Geometry: final body of the model. Coordinates: model frame, mm. Coordinates: 2 decimals unless noted, no trailing zeros. Order: outer loops, then holes, each group sorted by start corner. A loop starts at its lowest first (then second) coordinate and runs counter-clockwise, first axis right, second up. Notation, with made-up numbers: (-24, 12.5) -> (-12, 12.5) arc R26 ccw to (-12, 39.5) -> close; hole circle Ø11 at (-26, 26.25). An arc over 180 degrees is marked (long way). Use one line per item in the form item = value.
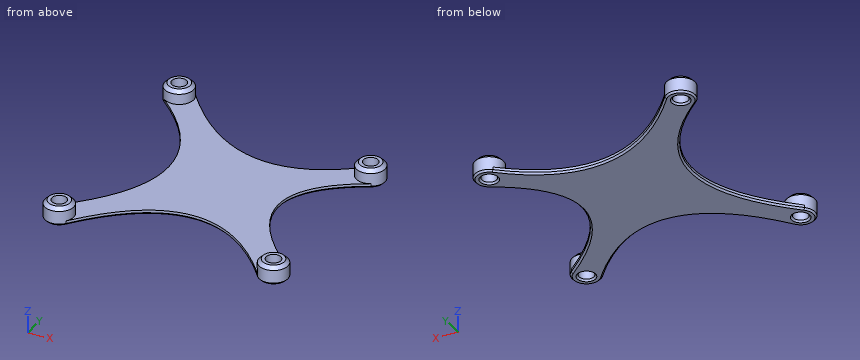
Autodesk Inventor part; units mm, degrees
ref_plane "YZ Plane" through (0, 0, 0) normal (1, 0, 0) x (0, 1, 0)
ref_plane "XZ Plane" through (0, 0, 0) normal (0, 1, 0) x (-1, 0, 0)
ref_plane "XY Plane" through (0, 0, 0) normal (0, 0, 1) x (1, 0, 0)
sketch "Skizze1" plane through (0, 0, 0) normal (0, 0, 1) x (1, 0, 0)
  circle A0 centre (-25.837, 27.4295) radius 1.65
  line L0 (-38.2086, 5.3216) -> (-37.4869, 5.3204)
  line L1 (-37.4869, 5.3204) -> (-37.4918, 2.4829)
  line L2 (-37.4918, 2.4829) -> (-35.7716, 2.4799)
  line L3 (-35.7716, 2.4799) -> (-35.7668, 5.1987)
  line L4 (-35.7668, 5.1987) -> (-35.0451, 5.1975)
  line L5 (-35.0451, 5.1975) -> (-35.0499, 2.4787)
  line L6 (-35.0499, 2.4787) -> (-32.1136, 2.4735)
  line L7 (-32.1136, 2.4735) -> (-32.115, 1.6628)
  line L8 (-32.115, 1.6628) -> (-38.215, 1.6735)
  line L9 (-38.215, 1.6735) -> (-38.2086, 5.3216)
  line L10 (-35.0952, -3.6509) -> (-32.1243, -3.6561)
  line L11 (-32.1243, -3.6561) -> (-32.1256, -4.4273)
  line L12 (-32.1256, -4.4273) -> (-34.7356, -4.4227)
  spline S0 degree 2 poles (-34.7356, -4.4227) (-35.052, -4.4222) (-35.5959, -4.4805) (-35.7592, -4.5692) knots 0 0 0 1 2 2 2
  spline S1 degree 2 poles (-35.7592, -4.5692) (-35.9323, -4.6628) (-36.101, -4.9987) (-36.1015, -5.2854) knots 0 0 0 1 2 2 2
  spline S2 degree 2 poles (-36.1015, -5.2854) (-36.102, -5.5721) (-35.7966, -6.1807) (-35.5499, -6.4728) knots 0 0 0 1 2 2 2
  line L13 (-35.5499, -6.4728) -> (-32.1292, -6.4787)
  line L14 (-32.1292, -6.4787) -> (-32.1305, -7.2499)
  line L15 (-32.1305, -7.2499) -> (-36.708, -7.2419)
  line L16 (-36.708, -7.2419) -> (-36.7066, -6.4707)
  line L17 (-36.7066, -6.4707) -> (-36.1975, -6.4716)
  spline S3 degree 2 poles (-36.1975, -6.4716) (-36.5083, -6.125) (-36.8334, -5.4571) (-36.8327, -5.0815) knots 0 0 0 1 2 2 2
  spline S4 degree 2 poles (-36.8327, -5.0815) (-36.8316, -4.4092) (-35.9405, -3.6495) (-35.0952, -3.6509) knots 0 0 0 1 2 2 2
  line L18 (-36.71, -8.3739) -> (-32.1325, -8.3819)
  line L19 (-32.1325, -8.3819) -> (-32.1338, -9.153)
  line L20 (-32.1338, -9.153) -> (-36.7113, -9.145)
  line L21 (-36.7113, -9.145) -> (-36.71, -8.3739)
  line L22 (-32.1384, -11.773) -> (-32.1398, -12.5837)
  line L23 (-32.1398, -12.5837) -> (-37.5181, -12.5743)
  line L24 (-37.5181, -12.5743) -> (-37.5217, -14.6208)
  line L25 (-37.5217, -14.6208) -> (-38.2434, -14.6195)
  line L26 (-38.2434, -14.6195) -> (-38.2348, -9.7158)
  line L27 (-38.2348, -9.7158) -> (-37.5131, -9.7171)
  line L28 (-37.5131, -9.7171) -> (-37.5167, -11.7636)
  line L29 (-37.5167, -11.7636) -> (-32.1384, -11.773)
  line L30 (-38.2719, -8.3168) -> (-37.4711, -8.3182)
  line L31 (-37.4711, -8.3182) -> (-37.4727, -9.1931)
  line L32 (-37.4727, -9.1931) -> (-38.2735, -9.1917)
  line L33 (-38.2735, -9.1917) -> (-38.2719, -8.3168)
  line L34 (-36.695, 0.2274) -> (-36.6936, 1.0282)
  line L35 (-36.6936, 1.0282) -> (-30.4347, -1.4445)
  line L36 (-30.4347, -1.4445) -> (-30.4362, -2.27)
  line L37 (-30.4362, -2.27) -> (-32.3428, -1.4461)
  line L38 (-32.3428, -1.4461) -> (-36.7008, -3.0994)
  line L39 (-36.7008, -3.0994) -> (-36.6993, -2.269)
  line L40 (-36.6993, -2.269) -> (-33.306, -1.0242)
  line L41 (-33.306, -1.0242) -> (-36.695, 0.2274)
  line L42 (-32.103, 8.529) -> (-32.5874, 8.5299)
  spline S5 degree 2 poles (-32.5874, 8.5299) (-32.5184, 8.4358) (-32.2718, 8.119) (-32.1979, 7.9706) knots 0 0 0 1 2 2 2
  spline S6 degree 2 poles (-32.1979, 7.9706) (-32.0895, 7.7677) (-31.9765, 7.3869) (-31.9771, 7.0409) knots 0 0 0 1 2 2 2
  spline S7 degree 2 poles (-31.9771, 7.0409) (-31.9775, 6.7591) (-32.191, 6.2503) (-32.3841, 6.0579) knots 0 0 0 1 2 2 2
  spline S8 degree 2 poles (-32.3841, 6.0579) (-32.5723, 5.8753) (-33.1263, 5.6538) (-33.4328, 5.6544) knots 0 0 0 1 2 2 2
  spline S9 degree 2 poles (-33.4328, 5.6544) (-33.9074, 5.6552) (-34.5789, 6.0568) (-34.771, 6.4921) knots 0 0 0 1 2 2 2
  spline S10 degree 2 poles (-34.771, 6.4921) (-34.9483, 6.878) (-35.0799, 7.9262) (-35.1134, 8.5343) knots 0 0 0 1 2 2 2
  line L43 (-35.1134, 8.5343) -> (-35.2617, 8.5345)
  spline S11 degree 2 poles (-35.2617, 8.5345) (-35.5287, 8.535) (-35.8602, 8.3725) (-35.9543, 8.2243) knots 0 0 0 1 2 2 2
  spline S12 degree 2 poles (-35.9543, 8.2243) (-36.0485, 8.0762) (-36.1086, 7.6512) (-36.109, 7.4238) knots 0 0 0 1 2 2 2
  spline S13 degree 2 poles (-36.109, 7.4238) (-36.1094, 7.1569) (-35.9525, 6.4349) (-35.7999, 6.0737) knots 0 0 0 1 2 2 2
  line L44 (-35.7999, 6.0737) -> (-35.8, 6.0292)
  line L45 (-35.8, 6.0292) -> (-36.586, 6.0306)
  spline S14 degree 2 poles (-36.586, 6.0306) (-36.6449, 6.2433) (-36.7918, 7.0394) (-36.7911, 7.4299) knots 0 0 0 1 2 2 2
  spline S15 degree 2 poles (-36.7911, 7.4299) (-36.7903, 7.9045) (-36.6409, 8.5518) (-36.4476, 8.8085) knots 0 0 0 1 2 2 2
  spline S16 degree 2 poles (-36.4476, 8.8085) (-36.2594, 9.0603) (-35.6608, 9.3064) (-35.2307, 9.3056) knots 0 0 0 1 2 2 2
  line L46 (-35.2307, 9.3056) -> (-32.1016, 9.3002)
  line L47 (-32.1016, 9.3002) -> (-32.103, 8.529)
  line L48 (-35.0644, 13.9817) -> (-32.0935, 13.9765)
  line L49 (-32.0935, 13.9765) -> (-32.0948, 13.2054)
  line L50 (-32.0948, 13.2054) -> (-34.7049, 13.2099)
  spline S17 degree 2 poles (-34.7049, 13.2099) (-35.0212, 13.2105) (-35.5651, 13.1521) (-35.7284, 13.0634) knots 0 0 0 1 2 2 2
  spline S18 degree 2 poles (-35.7284, 13.0634) (-35.9016, 12.9698) (-36.0702, 12.6339) (-36.0707, 12.3472) knots 0 0 0 1 2 2 2
  spline S19 degree 2 poles (-36.0707, 12.3472) (-36.0712, 12.0605) (-35.7658, 11.452) (-35.5191, 11.1599) knots 0 0 0 1 2 2 2
  line L51 (-35.5191, 11.1599) -> (-32.0984, 11.1539)
  line L52 (-32.0984, 11.1539) -> (-32.0998, 10.3828)
  line L53 (-32.0998, 10.3828) -> (-36.6772, 10.3907)
  line L54 (-36.6772, 10.3907) -> (-36.6759, 11.1619)
  line L55 (-36.6759, 11.1619) -> (-36.1667, 11.161)
  spline S20 degree 2 poles (-36.1667, 11.161) (-36.4775, 11.5076) (-36.8026, 12.1755) (-36.802, 12.5512) knots 0 0 0 1 2 2 2
  spline S21 degree 2 poles (-36.802, 12.5512) (-36.8008, 13.2235) (-35.9097, 13.9832) (-35.0644, 13.9817) knots 0 0 0 1 2 2 2
  circle A1 centre (-25.837, -24.3815) radius 1.65
  circle A2 centre (22.931, 18.2855) radius 1.65
  circle A3 centre (23.297, -24.3815) radius 1.65
  arc A4 (-37.7973, 28.9208) -> (-39.6082, 27.5864) centre (-37.7217, 26.9222) ccw
  arc A5 (-39.6082, 27.5864) -> (-39.8919, 25.917) centre (-34.8919, 25.926) ccw
  line L56 (-39.8919, 25.917) -> (-39.8874, 23.4424)
  line L57 (-39.8874, 23.4424) -> (-39.478, 23.4424)
  arc A6 (-39.478, 21.4424) -> (-39.478, 23.4424) centre (-34.8856, 22.4424) ccw
  line L58 (-39.478, 21.4424) -> (-39.8838, 21.4424)
  line L59 (-39.8838, 21.4424) -> (-39.8061, -21.5576)
  line L60 (-39.8061, -21.5576) -> (-39.3966, -21.5576)
  arc A7 (-39.3966, -23.5576) -> (-39.3966, -21.5576) centre (-34.8043, -22.5576) ccw
  line L61 (-39.3966, -23.5576) -> (-39.8025, -23.5576)
  line L62 (-39.8025, -23.5576) -> (-39.798, -26.0503)
  arc A8 (-39.798, -26.0503) -> (-39.5082, -27.7186) centre (-34.798, -26.0413) ccw
  arc A9 (-39.5082, -27.7186) -> (-37.6925, -29.0465) centre (-37.6241, -27.0477) ccw
  line L63 (-37.6925, -29.0465) -> (-31.8925, -29.036)
  spline S22 degree 2 poles (-31.8925, -29.036) (-30.8606, -29.0341) (-25.3454, -28.3512) knots -2 -2 -2 -1 -1 -1
  arc A10 (-25.3454, -28.3512) -> (-22.6346, -26.7782) centre (-25.837, -24.3815) ccw
  spline S23 degree 2 poles (-22.6346, -26.7782) (-1.453, 1.524) (20.1144, -26.8045) knots -2 -2 -2 -1 -1 -1
  arc A11 (20.1144, -26.8045) -> (25.8626, -21.3127) centre (23.297, -24.3815) ccw
  arc A12 (24.7305, 14.7131) -> (20.2403, 21.2453) centre (22.931, 18.2855) ccw
  spline S24 degree 2 poles (20.2403, 21.2453) (-1.453, 1.524) (-22.6346, 29.8262) knots -2 -2 -2 -1 -1 -1
  arc A13 (-22.6346, 29.8262) -> (-27.9876, 30.8022) centre (-25.837, 27.4295) ccw
  spline S25 degree 2 poles (-27.9876, 30.8022) (-30.9185, 28.9332) (-31.9973, 28.9313) knots -2 -2 -2 -1 -1 -1
  line L64 (-31.9973, 28.9313) -> (-37.7973, 28.9208)
  circle A14 centre (-25.837, 27.4295) radius 1.7
  circle A15 centre (-25.837, -24.3815) radius 1.7
  circle A16 centre (23.297, -24.3815) radius 1.7
  circle A17 centre (22.931, 18.2855) radius 1.7
  circle A18 centre (-25.837, 27.4295) radius 3.3
  circle A19 centre (22.931, 18.2855) radius 3.3
  circle A20 centre (23.297, -24.3815) radius 3.3
  circle A21 centre (-25.837, -24.3815) radius 3.3
  line L65 (-28.0198, -21.9065) -> (-1.453, 1.524) construction
  line L66 (-1.453, 1.524) -> (-28.0198, 24.9545) construction
  spline S26 degree 2 poles (-28.0198, -21.9065) (-1.453, 1.524) (-28.0198, 24.9545) knots 1 1 1 2 2 2
  line L67 (-23.2346, 29.4587) -> (-1.453, 1.524) construction
  line L68 (-1.453, 1.524) -> (20.77, 20.7795) construction
  spline S27 degree 2 poles (-23.2346, 29.4587) (-1.453, 1.524) (20.77, 20.7795) knots 1 1 1 2 2 2
  line L69 (-23.2346, -26.4107) -> (-1.453, 1.524) construction
  line L70 (-1.453, 1.524) -> (20.7111, -26.4317) construction
  spline S28 degree 2 poles (-23.2346, -26.4107) (-1.453, 1.524) (20.7111, -26.4317) knots 1 1 1 2 2 2
  line L71 (25.4629, -21.8918) -> (-1.453, 1.524) construction
  line L72 (-1.453, 1.524) -> (24.4854, 15.3745) construction
  spline S29 degree 2 poles (25.4629, -21.8918) (-1.453, 1.524) (24.4854, 15.3745) knots 1 1 1 2 2 2
  spline S30 degree 2 poles (25.8626, -21.3127) (21.9132, -18.0109) (19.0822, -14.9107) knots -2 -2 -2 -1.855416 -1.855416 -1.855416
  spline S31 degree 2 poles (17.22, 9.815) (18.4126, 10.8679) (19.8732, 11.8725) knots 1.825455 1.825455 1.825455 1.896249 1.896249 1.896249
  spline S32 degree 2 poles (17.22, -12.7436) (6.6116, 0.4487) (17.22, 9.815) knots -1.804293 -1.804293 -1.804293 -1.174545 -1.174545 -1.174545
  spline S33 degree 2 poles (19.8732, 11.8725) (22.0139, 13.3447) (24.7305, 14.7131) knots -1.103751 -1.103751 -1.103751 -1 -1 -1
  spline S34 degree 2 poles (19.0822, -14.9107) (18.0812, -13.8146) (17.22, -12.7436) knots 1.144584 1.144584 1.144584 1.195707 1.195707 1.195707
  point P0 (0, 0)
  point P1 (24.4854, 15.3745)
  point P2 (20.77, 20.7795)
  dimension "d5" = 6.6
  dimension "d0" = 3.4
  dimension "d1" = 3.4
  dimension "d2" = 3.4
  dimension "d3" = 3.4
  dimension "d4" = 1.6
  dimension "d6" = 6.6
  dimension "d7" = 6.6
  dimension "d8" = 6.6
  dimension "d9" = 51.811
  dimension "d10" = 25.9055
  dimension "d11" = 48.768
  dimension "d12" = 24.384
extrude "Extrusion1" add sketch "Skizze1" along normal blind 1 contours A18 | A18 S27 A19 S29 A20 S28 A21 S26 | A19 | A21 | A20
sketch "Skizze2" plane through (0, 0, 1) normal (0, 0, 1) x (1, 0, 0)
  circle A0 centre (-25.837, 27.4295) radius 1.7
  circle A1 centre (22.931, 18.2855) radius 1.7
  circle A2 centre (23.297, -24.3815) radius 1.7
  circle A3 centre (-25.837, -24.3815) radius 1.7
  circle A4 centre (-25.837, 27.4295) radius 1.7
  circle A5 centre (-25.837, 27.4295) radius 3.3
  circle A6 centre (22.931, 18.2855) radius 3.3
  circle A7 centre (23.297, -24.3815) radius 3.3
  circle A8 centre (-25.837, -24.3815) radius 3.3
  point P0 (0, 0)
  dimension "d15" = 6.6
  dimension "d16" = 6.6
  dimension "d17" = 6.6
  dimension "d18" = 6.6
extrude "Extrusion2" add sketch "Skizze2" along normal blind 3.2
chamfer "Fase1" distance 0.4 angle 45 12 edges at (-1.3426, 13.3215, 0) (-28.0988, 29.8325, 0) (-14.7364, 1.524, 0) (-28.0988, -26.7845, 0) (-1.3574, -12.4486, 0) (25.5766, -26.7676, 0) (11.7606, -0.8673, 0) (25.6505, 20.1549, 0) (-27.537, 27.4295, 0) (-27.537, -24.3815, 0) (21.597, -24.3815, 0) (21.231, 18.2855, 0)
chamfer "Fase2" distance 0.8 angle 45 4 edges at (-29.137, 27.4295, 4.2) (19.631, 18.2855, 4.2) (19.997, -24.3815, 4.2) (-29.137, -24.3815, 4.2)
equation "\"d6\" = d5"
equation "\"d7\" = d5"
equation "\"d8\" = d5"
equation "\"d10\" = 0.5 * d9"
equation "\"d12\" = 0.5 * d11"
properties part number "TinyFan_Extrusion_Top"
1) Section A-A, the plane z = 2. Output: boundary loops of the cut face in (x, y), and give its area (3 significant figures).
Results found:
outline = circle Ø6.6 at (-25.84, -24.38); circle Ø6.6 at (-25.84, 27.43); circle Ø6.6 at (22.93, 18.29); circle Ø6.6 at (23.3, -24.38); hole circle Ø3.4 at (-25.84, -24.38); hole circle Ø3.4 at (-25.84, 27.43); hole circle Ø3.4 at (22.93, 18.29); hole circle Ø3.4 at (23.3, -24.38)
area = 101 mm2
2) Material intervals for probe 1 along X at (y, z) = (18, 0.8); probe 2 along Z at (x, y) = (-25, 23.5); probe 3 along Y at (x, z) = (-23.5, 3.85), sorted ascending. Write a range as from..to.
Results found:
probe_1 = -21.3..-11.71, 17.22..21.26, 24.61..26.22
probe_2 = 0..1
probe_3 = -26.01..-22.75, 25.8..29.06
3) Contact query for flat-ended pins moving along their axis: P1, Ø4, axis at x = -25.84, y = -24.38, coming from the +Z side; P2, Ø3, axis at x = -14.5, y = 6.5, coming from the +Z side; P3, Ø1.5, axis at x = -1.5, z = 1, coming from the +Y side. Output: stop coordinate, or through.
Results found:
P1 = 4.2
P2 = 1
P3 = 13.52
